Source: CAD feature listing. Evaluate the final solid. Frame: model axes, mm. A direction names the side the tool comes from. Coordinates: 2 decimals unless noted, no trailing zeros. Loops run counter-clockwise (first coordinate to the right, second up) from the corner with the lowest first, then second, coordinate; pieces in that order, holes last. Notation, with made-up numbers: (-22.75, 2) - (22.25, 2) arc R24 ccw to (22.25, 15) - close; hole circle Ø9 at (30.5, 51.25). An arc over 180 degrees is marked (long way). Write item = value, one per line. Start each with the question number.
Autodesk Fusion 360 part; units mm, degrees
sketch "Boceto2" plane through (0, 4, 0) normal (0, 1, 0) x (-1, 0, 0)
  line L0 (9, 0) -> (-1, 0)
  line L1 (-30, 0) -> (-60, 0)
  line L2 (-30, 0) -> (0, 0)
  line L3 (-30, 25) -> (-30, -10)
  line L4 (-30, -10) -> (-60, -10)
  line L5 (-60, -10) -> (-60, 60)
  line L6 (-60, 60) -> (0, 60)
  line L7 (0, 60) -> (0, -10)
  line L8 (0, -10) -> (-30, -10)
  line L9 (0, -10) -> (-5, -10)
  line L10 (-5, -10) -> (-5, -5)
  line L11 (-5, -5) -> (-55, -5)
  line L12 (-55, -5) -> (-55, 55)
  line L13 (-55, 55) -> (-5, 55)
  line L14 (-5, 55) -> (-5, -5)
  dimension "d1" = 10
  dimension "d2" = 30
  dimension "d3" = 30
  dimension "d4" = 35
  dimension "d5" = 70
  dimension "d6" = 5
  dimension "d7" = 5
  dimension "d8" = 50
  dimension "d9" = 60
extrude "Extruir1" add sketch "Boceto2" along normal blind 20 contours L0 L2 L7 L8 L9 L10 L14 | L0 L1 L2 L5 L6 L7 L12 L13 L14 | L3 L8 L10 L11 | L1 L3 L4 L5 L11 L12
sketch "Boceto3" plane through (0, 4, 0) normal (0, 1, 0) x (-1, 0, 0)
  line L0 (0, -10) -> (-5, -10)
  line L1 (-5, -10) -> (-10, -20)
  line L2 (0, -10) -> (0, -20)
  line L3 (0, -20) -> (-60, -20)
  line L4 (-60, -20) -> (-60, -10)
  line L5 (-60, -10) -> (-64.5056, 6.5239)
  line L6 (0, 60) -> (0, 70)
  line L7 (0, 70) -> (-60, 70)
  line L8 (-60, 70) -> (-60, 60)
  line L9 (-60, 60) -> (0, 60)
  line L10 (-5, -10) -> (-60, -10)
  dimension "d12" = 10
  dimension "d13" = 10
extrude "Extruir2" add sketch "Boceto3" along normal blind 4
sketch "Boceto4" plane through (0, 8, 0) normal (0, 1, 0) x (-1, 0, 0)
  line L0 (0, -10) -> (-60, -10)
  line L1 (-60, -10) -> (-60, -20)
  line L2 (-60, -20) -> (0, -20)
  line L3 (0, -20) -> (0, -10)
  line L4 (0, -15) -> (-20, -15)
  line L5 (-26, -15) -> (-35, -15)
  line L6 (-20, -15) -> (-40, -15)
  line L7 (-40, -15) -> (-80, 70)
  line L8 (0, 70) -> (0, 65)
  line L9 (0, 65) -> (-20, 65)
  line L10 (-20, 65) -> (-40, 65)
  circle A0 centre (-40, 65) radius 1.5
  circle A1 centre (-20, 65) radius 1.5
  circle A2 centre (-20, -15) radius 1.5
  circle A3 centre (-40, -15) radius 1.5
  dimension "d16" = 20
  dimension "d17" = 3
  dimension "d18" = 3
  dimension "d19" = 3
  dimension "d20" = 3
extrude "Extruir3" cut sketch "Boceto4" against normal blind 30 contours L6 L7 A3 | L6 L7 A3 | L4 L6 A2 | L4 L6 A2 | L9 L10 A1 | L9 L10 A1 | A0
sketch "Boceto5" plane through (0, 24, 0) normal (0, 1, 0) x (-1, 0, 0)
  line L0 (-55, 55) -> (-5, 55)
  line L1 (-5, 55) -> (-5, -5)
  line L2 (-5, -5) -> (-55, -5)
  line L3 (-55, -5) -> (-55, 55)
  line L4 (0, -10) -> (0, 60)
  line L5 (0, 60) -> (-60, 60)
  line L6 (-60, 60) -> (-60, -10)
  line L7 (-60, -10) -> (0, -10)
  line L8 (0, -10) -> (-60, -10)
  line L9 (-60, 60) -> (-60, -10)
  line L10 (-60, 60) -> (0, 60)
  line L11 (0, -8.1337) -> (20, 20)
  line L12 (0, -10) -> (0, 60)
extrude "Extruir4" add sketch "Boceto5" along normal blind 2 contours L0 L1 L2 L3 | L4 L5 L6 L7 L8 L9 L10 L12
sketch "Boceto6" plane through (60, 0, 0) normal (1, 0, 0) x (0, 0, -1)
  line L0 (-70, 4) -> (20, 4)
  line L1 (20, 4) -> (20, 8)
  line L2 (20, 8) -> (10, 8)
  line L3 (10, 8) -> (10, 26)
  line L4 (10, 26) -> (-60, 26)
  line L5 (-60, 26) -> (-60, 8)
  line L6 (-60, 8) -> (-70, 8)
  line L7 (-70, 8) -> (-70, 4)
sketch "Boceto7" plane through (0, 4, 0) normal (0, -1, 0) x (1, 0, 0)
  circle A0 centre (40, -15) radius 1.5
  circle A1 centre (20, 65) radius 1.5
  circle A2 centre (20, -15) radius 1.5
  circle A3 centre (40, 65) radius 1.5
  line L0 (5, 55) -> (55, 55)
  line L1 (55, 55) -> (55, -5)
  line L2 (55, -5) -> (5, -5)
  line L3 (5, -5) -> (5, 55)
  line L4 (0, 70) -> (0, -20)
  line L5 (0, -20) -> (60, -20)
  line L6 (60, -20) -> (60, 70)
  line L7 (60, 70) -> (0, 70)
  line L8 (5, 55) -> (0, 55)
  line L9 (5, -5) -> (0, -5)
  line L10 (0, 55) -> (0, -5)
  line L11 (5, 55) -> (5, -5)
  line L12 (55, 55) -> (60, 55)
  line L13 (60, 55) -> (60, -5)
  line L14 (55, -5) -> (60, -5)
  line L15 (55, -5) -> (55, 55)
extrude "Extruir5" cut sketch "Boceto7" against normal blind 20 contours L3 L4 L8 L9 L10 L11 | L1 L6 L12 L13 L14 L15
Item 1: Cut plane A-A (z = 65). Return the cut outline in (x, y).
Item 2: Cut plane D-D (x = 50). Return the cut outline in (y, z), then the cut area to 3 significant figures.
Item 3: Cut plane C-C (x = 40). Return the cut outline in (y, z).
Item 4: Material intervals for L1, parallel to Z at x = 20, y = 5.55; L2, parallel to X at y = 6.35, z = 65; L3, parallel to Z at x = 42.5, y = 16, sorted ascending. Write a range as [from, to].
Item 5: Reachability of faces 1 (the cylindrical face through (21.11, 6.03, 66.01)), 2 (the flat face through (30, 8, -15)), 3 (the flat face through (30, 24, 25)), 4 (the flat face through (30, 17, 60)) from +Z, -Z, +X, -X, +Y, -Y: full face, straight path, thin tool, end or side. Return the list, or none.
Item 6: Draft query along X for faces 5 (the flat face through (60, 25, 18)), 6 (the flat face through (30, 6, 70)), 7 (the cylindrical face through (41.5, 6.03, -14.93)). Return one class per face: released by +X, released by -X, zero draft, split by the parting line, or undercut.
Item 7: Cut plane B-B (y = 15). Return the cut outline in (x, z), then the cut area to 3 significant figures.
Item 8: First-contact query: pin 1 (4 mm diameter, centred on x = 40, z = -15, fed in from +Y); pin 2 (4 mm diameter, centred on x = 35.5, y = 10.5, fed in from -Z); pin 3 (10 mm diameter, centred on x = 31, z = 36.5, fed in from -Y). Flat tips, straight axial feed; report the tip coordinate or a pass-through.
Responses:
q1.outline = (0, 4) - (18.5, 4) - (18.5, 8) - (0, 8) - close; (21.5, 4) - (38.5, 4) - (38.5, 8) - (21.5, 8) - close; (41.5, 4) - (60, 4) - (60, 8) - (41.5, 8) - close
q2.outline = (4, -20) - (8, -20) - (8, -10) - (26, -10) - (26, 60) - (8, 60) - (8, 70) - (4, 70) - (4, 55) - (24, 55) - (24, -5) - (4, -5) - close
q2.area = 420 mm2
q3.outline = (4, -20) - (8, -20) - (8, -16.5) - (4, -16.5) - close; (4, -13.5) - (8, -13.5) - (8, -10) - (26, -10) - (26, 60) - (8, 60) - (8, 63.5) - (4, 63.5) - (4, 55) - (24, 55) - (24, -5) - (4, -5) - close; (4, 66.5) - (8, 66.5) - (8, 70) - (4, 70) - close
q4.L1 = [-20, -16.5], [-13.5, -5], [55, 63.5], [66.5, 70]
q4.L2 = [0, 18.5], [21.5, 38.5], [41.5, 60]
q4.L3 = [-10, -5], [55, 60]
q5.face_1 = +Y, -Y
q5.face_2 = -Z, +X, -X, +Y
q5.face_3 = +X, -X, -Y
q5.face_4 = +Z, +X, -X, +Y
q6.face_5 = released by +X
q6.face_6 = zero draft
q6.face_7 = undercut
q7.outline = (0, -10) - (60, -10) - (60, -5) - (0, -5) - close; (0, 55) - (60, 55) - (60, 60) - (0, 60) - close
q7.area = 600 mm2
q8.pin_1 = 8
q8.pin_2 = -10
q8.pin_3 = 24
